Input: part model. Units: mm. Frame: model coordinates. A direction names the side the tool comes from. Coordinates: 2 decimals unless noted, no trailing zeros. Put each result on its own line as item: value. Start each with the question number.
1. Pin query (flat end, axial travel): pin 1 (9 mm diameter, centred on x = 35.5, z = 11, fed in from +Y). Return the tip coordinate at first contact, or that it passes through.
2. Line query: line 1 (X direction, y = 39.5, z = 17.5); line 2 (X direction, y = 54, z = 13); line 3 (X direction, y = 36.5, z = 7.25). Output: solid intervals per line, ascending.
3. Access query for faces 5 (the flat face through (314, 60.5, 14)), 6 (the flat face through (31, 54.5, 10)), 7 (the flat face through (306, 31, 20)). Directions: +Z, -Z, +X, -X, +Y, -Y. A direction counts if a zero-diameter tool reaches every point of the face in a straight line with its end or side. Return the directions, or none.
4. Pull-direction query (X, two-part tool) for faces 1 (the flat face through (581, 54.5, 10)), 2 (the flat face through (306, 54.5, 10)), 3 (the flat face through (306, 0, 10)), 4 (the flat face through (620, 31, 10)); classes: released by +X, released by -X, zero draft, split by the parting line, or undercut.
from build123d import *

# Parameters (mm, degrees)
SKETCH_1_W                   = 620
SKETCH_1_H                   = 62
EXTRUDE_1_DEPTH              = 20
SKETCH_2_W                   = 12
SKETCH_2_H                   = 1.5
CUT_EXTRUDE_1_DEPTH          = 624.413185616
HOLE_WIZARD_M6_1_D           = 7
HOLE_WIZARD_M6_1_CBORE_D     = 11
HOLE_WIZARD_M6_1_CBORE_DEPTH = 6
HOLE_WIZARD_M3_1_D           = 2.5
HOLE_WIZARD_M3_1_DEPTH       = 7.5
HOLE_WIZARD_M3_1_TIP         = 0.751075774
HOLE_WIZARD_M3_2_D           = 2.5
HOLE_WIZARD_M3_2_DEPTH       = 7.5
HOLE_WIZARD_M3_2_TIP         = 0.751075774


with BuildPart() as part:
    # 草图1 → 凸台-拉伸1 (new body)
    with BuildSketch(Plane.XY):
        with Locations((310, 31)):
            Rectangle(SKETCH_1_W, SKETCH_1_H)
    extrude(amount=EXTRUDE_1_DEPTH)

    # 草图2 → 切除-拉伸1 (cut, through all)
    with BuildSketch(Plane(origin=(620, 0, 0), x_dir=(0, 0, -1), z_dir=(1, 0, 0))):
        with Locations((-10, 61.25)):
            Rectangle(SKETCH_2_W, SKETCH_2_H)
    extrude(amount=-CUT_EXTRUDE_1_DEPTH, mode=Mode.SUBTRACT)

    # M6 六角凹头螺钉的柱形沉头孔1 (through all)
    with Locations(Plane(origin=(0, 60.5, 0), x_dir=(-1, 0, 0), z_dir=(0, 1, 0))):
        with Locations((-35, 10), (-310, 10), (-585, 10)):
            CounterBoreHole(HOLE_WIZARD_M6_1_D / 2, HOLE_WIZARD_M6_1_CBORE_D / 2, HOLE_WIZARD_M6_1_CBORE_DEPTH)

    # M3 螺纹孔1
    with Locations(Plane(origin=(0, 60.5, 0), x_dir=(-1, 0, 0), z_dir=(0, 1, 0))):
        with Locations((-20, 10), (-445, 10), (-345, 10), (-245, 10), (-145, 10)):
            Hole(HOLE_WIZARD_M3_1_D / 2, depth=HOLE_WIZARD_M3_1_DEPTH)
            with Locations((0, 0, -(HOLE_WIZARD_M3_1_DEPTH + HOLE_WIZARD_M3_1_TIP / 2))):  # 118° drill point
                Cone(0, HOLE_WIZARD_M3_1_D / 2, HOLE_WIZARD_M3_1_TIP, mode=Mode.SUBTRACT)

    # M3 螺纹孔2
    with Locations(Plane.XY.offset(20)):
        with Locations((48.5, 39.5), (68, 39.5), (507, 39.5), (526.5, 39.5)):
            Hole(HOLE_WIZARD_M3_2_D / 2, depth=HOLE_WIZARD_M3_2_DEPTH)
            with Locations((0, 0, -(HOLE_WIZARD_M3_2_DEPTH + HOLE_WIZARD_M3_2_TIP / 2))):  # 118° drill point
                Cone(0, HOLE_WIZARD_M3_2_D / 2, HOLE_WIZARD_M3_2_TIP, mode=Mode.SUBTRACT)


solid = part.part
Report:
1. pin 1: stops at y = 60.5
2. line 1: x = 0 to 47.25, 49.75 to 66.75, 69.25 to 505.75, 508.25 to 525.25, 527.75 to 620
2. line 2: x = 0 to 33.2, 36.8 to 308.2, 311.8 to 583.2, 586.8 to 620
2. line 3: x = 0 to 32.83, 37.17 to 307.83, 312.17 to 582.83, 587.17 to 620
3. face 5: +X, -X, +Y
3. face 6: +Y
3. face 7: +Z, +X, -X, +Y, -Y
4. face 1: undercut
4. face 2: undercut
4. face 3: zero draft
4. face 4: released by +X
